from build123d import *

# Parameters (mm, degrees)
BOSS_EXTRUDE1_DEPTH = 3


with BuildPart() as part:
    # Sketch1 → Boss-Extrude1 (new body)
    with BuildSketch(Plane.XY):
        Polygon((25, 106), (20, 106), (20, 65.864378278), (5, 103), (5, 106), (0, 106), (0, 0), (5, 0), (5, 3), (20, 40.135621722), (20, 0), (25, 0), (25, 40.135621722), (40, 3), (40, 0), (45, 0), (45, 106), (40, 106), (40, 103), (25, 65.864378278), align=None)
        Polygon((40, 16.350215981), (25.196241916, 53), (40, 89.649784019), align=None, mode=Mode.SUBTRACT)
        Polygon((19.803758084, 53), (5, 16.350215981), (5, 89.649784019), align=None, mode=Mode.SUBTRACT)
    extrude(amount=BOSS_EXTRUDE1_DEPTH)


solid = part.part
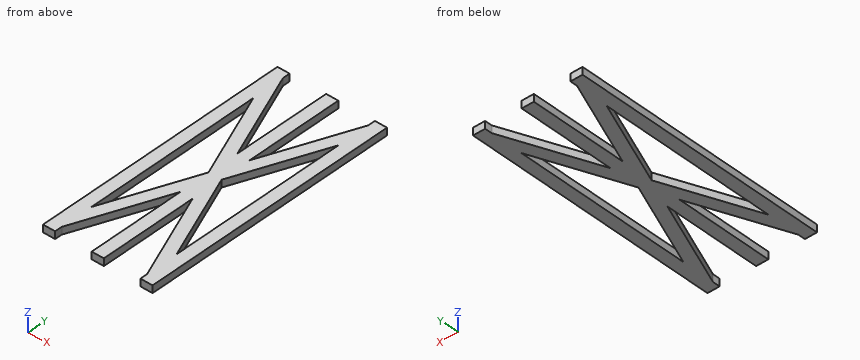
Geometry: final body of the model. Coordinates: model frame, mm. Give positions to 0.01 mm unless a question says otherwise; leave off trailing zeros. Write each loop counter-clockwise with the first axis right and the second up, starting at its lowest first coordinate (ties: lowest second). Pieces come first, ordered by that corner, then holes.
(1) First-contact query: P1, Ø1.5, axis at x = 7.5, z = 1.5, coming from the -Y side. Flat tip, straight axial feed; report the tip coordinate or a pass-through.
(2) Cut plane B-B, the plane y = 92.5. Return loops of the section in (x, z), then the cut area to 3 significant figures.
(3) Ray query, line 1 (X direction, y = 49.5, z = 1.6); line 2 (X direction, y = 24.5, z = 0.7); line 3 (X direction, y = 5.5, z = 0.55). Return the intervals inside material, ascending.
(4) Cut plane D-D, the plane y = 76. Return loops of the section in (x, z).
(5) Cut plane C-C, the plane x = 12. Return loops of the section in (y, z), then the cut area to 3 significant figures.
(6) Cut plane A-A, the plane z = 0.9. Return loops of the section in (x, y), then the cut area to 3 significant figures.
Values follow:
1. P1: stops at y = 7.33
2. outline: (0, 0) - (9.24, 0) - (9.24, 3) - (0, 3) - close; (20, 0) - (25, 0) - (25, 3) - (20, 3) - close; (35.76, 0) - (45, 0) - (45, 3) - (35.76, 3) - close
2. area: 70.4 mm2
3. line 1: x = 0 to 5, 18.39 to 26.61, 40 to 45
3. line 2: x = 0 to 5, 8.29 to 13.68, 20 to 25, 31.32 to 36.71, 40 to 45
3. line 3: x = 0 to 6.01, 20 to 25, 38.99 to 45
4. outline: (0, 0) - (5, 0) - (5, 3) - (0, 3) - close; (10.51, 0) - (15.91, 0) - (15.91, 3) - (10.51, 3) - close; (20, 0) - (25, 0) - (25, 3) - (20, 3) - close; (29.09, 0) - (34.49, 0) - (34.49, 3) - (29.09, 3) - close; (40, 0) - (45, 0) - (45, 3) - (40, 3) - close
5. outline: (20.33, 0) - (33.68, 0) - (33.68, 3) - (20.33, 3) - close; (72.32, 0) - (85.67, 0) - (85.67, 3) - (72.32, 3) - close
5. area: 80.1 mm2
6. outline: (0, 0) - (5, 0) - (5, 3) - (20, 40.14) - (20, 0) - (25, 0) - (25, 40.14) - (40, 3) - (40, 0) - (45, 0) - (45, 106) - (40, 106) - (40, 103) - (25, 65.86) - (25, 106) - (20, 106) - (20, 65.86) - (5, 103) - (5, 106) - (0, 106) - close; hole (5, 16.35) - (19.8, 53) - (5, 89.65) - close; hole (25.2, 53) - (40, 16.35) - (40, 89.65) - close
6. area: 2,390 mm2
